```python
from build123d import *

# Parameters (mm, degrees)
SKETCH_1_R          = 5
EXTRUDE_1_DEPTH     = 69.1
SKETCH_3_R          = 4
EXTRUDE_3_DEPTH     = 15
CUT_EXTRUDE_1_DEPTH = 1.8


with BuildPart() as part:
    # ｽｹｯﾁ1 → ﾎﾞｽ - 押し出し1 (new body)
    with BuildSketch(Plane.XY):
        Circle(SKETCH_1_R)
    extrude(amount=EXTRUDE_1_DEPTH)

    # ｽｹｯﾁ3 → ﾎﾞｽ - 押し出し3 (add)
    with BuildSketch(Plane(origin=(0, 0, 0), x_dir=(-1, 0, 0), z_dir=(0, 0, -1))):
        Circle(SKETCH_3_R)
    extrude(amount=EXTRUDE_3_DEPTH)

    # ｽｹｯﾁ4 → ｶｯﾄ - 押し出し1 (cut)
    with BuildSketch(Plane(origin=(0, 5, 0), x_dir=(1, 0, 0), z_dir=(0, 1, 0))):
        with BuildLine():
            ThreePointArc((1.5, -54.1), (0, -52.6), (-1.5, -54.1))
            Line((-1.5, -54.1), (1.5, -54.1))
        make_face()
        with BuildLine():
            Line((1.5, -54.1), (-1.5, -54.1))
            ThreePointArc((-1.5, -54.1), (0, -55.6), (1.5, -54.1))
        make_face()
        with BuildLine():
            ThreePointArc((1.5, -54.1), (0, -55.6), (-1.5, -54.1))
            Line((-1.5, -54.1), (-1.5, -69.1))
            Line((-1.5, -69.1), (1.5, -69.1))
            Line((1.5, -69.1), (1.5, -54.1))
        make_face()
    extrude(amount=-CUT_EXTRUDE_1_DEPTH, mode=Mode.SUBTRACT)


solid = part.part
```
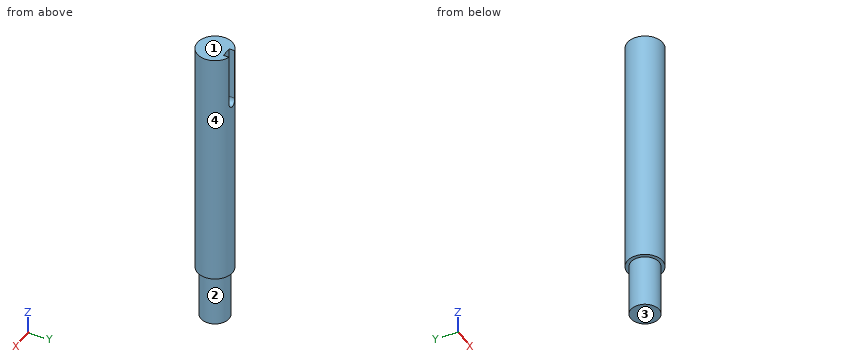
Check sheet for the modelled part. Datum: model origin and axes. Units: mm. Face numbers are marked on the shaded views. A direction names the side the tool comes from. Coordinates: 2 decimals unless noted, no trailing zeros. Loops run counter-clockwise (first coordinate to the right, second up) from the corner with the lowest first, then second, coordinate; pieces in that order, holes last.
1) Material ranges on probe 1 along X at (y, z) = (-3, 48.5); probe 2 along Z at (x, y) = (2.25, 3.5), recorded low to high.
2) Sectioned sample at A-A (x = 0). Record the boundary of the cut face in (y, z).
3) Gauge pin test, flat ends, axial feed: pin 1 (3.5 mm diameter, centred on x = -0.5, z = 64, fed in from +Y); pin 2 (6 mm diameter, centred on x = -1, z = 35.5, fed in from -Y); pin 3 (3 mm diameter, centred on y = 2.5, z = 9, fed in from -X); pin 4 (0.8 mm diameter, centred on y = 3.5, z = 60, fed in from -X). Record the tip position at first contact, or that the pin passes through.
4) Sectioned sample at C-C (z = 58). Record the boundary of the cut face in (x, y).
5) Access from +Z, -Z, +X, -X, +Y, -Y to the whole of each face (thin tool, end or side, straight path). Record for the marked faces 1 and 2.
6) Sectioned sample at B-B (y = 0). Record the boundary of the cut face in (x, z), and give its area (3 significant figures).
7) Release check for a two-part mould opening along Y. For the marked faces 3 and 4 record: released by +Y, released by -Y, zero draft, split by the parting line, or undercut.
8) Sectioned sample at D-D (y = -3). Record the boundary of the cut face in (x, z).
Check sheet entries:
1. probe 1: x = -4 to 4
1. probe 2: z = 0 to 69.1
2. outline: (-5, 0) - (-4, 0) - (-4, -15) - (4, -15) - (4, 0) - (5, 0) - (5, 52.6) - (3.2, 52.6) - (3.2, 69.1) - (-5, 69.1) - close
3. pin 1: stops at y = 4.77
3. pin 2: stops at y = -5
3. pin 3: stops at x = -4.9
3. pin 4: stops at x = -3.92
4. outline: (-1.5, 3.2) - (-1.5, 4.77) arc R5 ccw (long way) to (1.5, 4.77) - (1.5, 3.2) - close
5. face 1: +Z, +X, -X, +Y, -Y
5. face 2: -Z
6. outline: (-5, 0) - (-4, 0) - (-4, -15) - (4, -15) - (4, 0) - (5, 0) - (5, 69.1) - (-5, 69.1) - close
6. area: 811 mm2
7. face 3: zero draft
7. face 4: split by the parting line
8. outline: (-4, 0) - (-2.65, 0) - (-2.65, -15) - (2.65, -15) - (2.65, 0) - (4, 0) - (4, 69.1) - (-4, 69.1) - close
